Could you check a few things on this model? Use its own coordinates, in mm. Give positions to 0.01 mm unless a question says otherwise; leave off trailing zeros. Order: outer loops, then holes, each group sorted by start corner. A loop starts at its lowest first (then second) coordinate and runs counter-clockwise, first axis right, second up.
(1) Imagine slicing it at A-A, the plane y = -44. Write out the boundary of the cut face in (x, z) (3 decimals).
(2) Imagine slicing it at D-D, the plane x = 0. Write out the boundary of the cut face in (y, z) (3 decimals).
(3) Will these pins go through, and if not, where does the flat tip stop? pin 1 (8 mm diameter, centred on x = 62.27, y = -12.45, fed in from -Z); pin 2 (1 mm diameter, centred on x = 28.5, z = 2, fed in from +Y); pin 3 (1 mm diameter, centred on x = 58.5, z = 1.5, fed in from -Y).
(4) Imagine slicing it at B-B, the plane x = 61.5. Write out the boundary of the cut face in (y, z) (3 decimals), then the cut area to 3 significant figures.
(5) Imagine slicing it at C-C, the plane z = 0.5. Write out the boundary of the cut face in (x, y).
(6) If I drill on probe 1 along X at (y, z) = (-11, 1.05); probe 2 along X at (y, z) = (-12, 1.6); probe 3 along Y at (x, z) = (0, 2.5), over which ranges is the centre line in solid material (lowest first)?
from build123d import *

# Parameters (mm, degrees)
BOSS_EXTRUDE1_DEPTH     = 3.175
F_1_4_20_TAPPED_HOLE1_D = 5.1054


with BuildPart() as part:
    # Sketch1 → Boss-Extrude1 (new body)
    with BuildSketch(Plane.XY):
        with BuildLine():
            ThreePointArc((-50.528450834, 57.037844072), (-37.969184963, -66.066489185), (74.720247488, -14.944049498))
            ThreePointArc((74.720247488, -14.944049498), (64.757547823, 0), (49.813498325, -9.962699665))
            ThreePointArc((49.813498325, -9.962699665), (-25.312789976, -44.044326123), (-33.685633889, 38.025229381))
            ThreePointArc((-33.685633889, 38.025229381), (-32.600735016, 55.952945199), (-50.528450834, 57.037844072))
        make_face()
    extrude(amount=BOSS_EXTRUDE1_DEPTH)

    # 1/4-20 Tapped Hole1 (through all)
    with Locations(Plane.XY.offset(3.175)):
        with Locations((62.266872906, -12.453374581)):
            Hole(F_1_4_20_TAPPED_HOLE1_D / 2)


solid = part.part
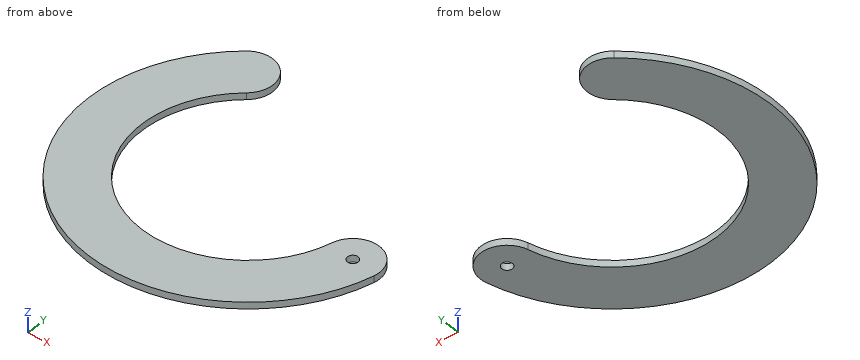
Answer block:
1. outline: (-62.213, 0) - (-25.39, 0) - (-25.39, 3.175) - (-62.213, 3.175) - close; (25.39, 0) - (62.213, 0) - (62.213, 3.175) - (25.39, 3.175) - close
2. outline: (-76.2, 0) - (-50.8, 0) - (-50.8, 3.175) - (-76.2, 3.175) - close
3. pin 1: stops at z = 0
3. pin 2: stops at y = -41.71
3. pin 3: stops at y = -49.42
4. outline: (-44.991, 0) - (-14.888, 0) - (-14.888, 3.175) - (-44.991, 3.175) - close; (-10.019, 0) - (0.223, 0) - (0.223, 3.175) - (-10.019, 3.175) - close
4. area: 128 mm2
5. outline: (-50.53, 57.04) arc R76.2 ccw (long way) to (74.72, -14.94) arc R12.7 ccw to (49.81, -9.96) arc R50.8 cw (long way) to (-33.69, 38.03) arc R12.7 ccw to start; hole circle Ø5.11 at (62.27, -12.45)
6. probe 1: x = -75.4 to -49.59, 49.59 to 60.17, 64.37 to 74.88
6. probe 2: x = -75.25 to -49.36, 49.36 to 59.75, 64.78 to 74.96
6. probe 3: y = -76.2 to -50.8
